Part model, mm, in its own coordinate system. A direction names the side the tool comes from. Coordinates: 2 decimals unless noted, no trailing zeros. Write each loop counter-clockwise with the first axis right and the second up, starting at its lowest first coordinate (ties: lowest second). Pieces come first, ordered by that corner, then holes. Notation, with made-up numbers: (-36.75, 70) - (14.25, 70) arc R19 cw to (14.25, 87) - close; hole circle Ø7 at (25, -20.5). An arc over 180 degrees is marked (long way). Use a Markdown table: item, result.
```python
from build123d import *

# Parameters (mm, degrees)
F0_R     = 7.9375
F0_R_2   = 11.828435
F0_R_3   = 12.7
F0_R_4   = 6.35
F1_DEPTH = 12.7


with BuildPart() as f1:
    # F0 (on Front) → F1 (new body)
    with BuildSketch(Plane.XZ):
        with BuildLine():
            Line((82.55, 7.45639), (82.55, 34.925))
            ThreePointArc((82.55, 34.925), (50.8, 66.675), (19.05, 34.925))
            Line((19.05, 34.925), (19.05, 33.3375))
            ThreePointArc((19.05, 33.3375), (17.655096, 29.969904), (14.2875, 28.575))
            Line((14.2875, 28.575), (-14.2875, 28.575))
            ThreePointArc((-14.2875, 28.575), (-17.655096, 29.969904), (-19.05, 33.3375))
            Line((-19.05, 33.3375), (-19.05, 34.925))
            ThreePointArc((-19.05, 34.925), (-50.8, 66.675), (-82.55, 34.925))
            Line((-82.55, 34.925), (-82.55, 7.45639))
            ThreePointArc((-82.55, 7.45639), (-83.623483, 4.44432), (-86.36, 2.790112))
            ThreePointArc((-86.36, 2.790112), (-101.503534, -17.789696), (-82.55, -34.925))
            Line((-82.55, -34.925), (-53.975, -34.925))
            ThreePointArc((-53.975, -34.925), (-47.239808, -37.714808), (-44.45, -44.45))
            Line((-44.45, -44.45), (-44.45, -51.575074))
            ThreePointArc((-44.45, -51.575074), (-41.660192, -58.310266), (-34.925, -61.100074))
            Line((-34.925, -61.100074), (-18.634955, -61.100074))
            Line((-18.634955, -61.100074), (-18.634955, -48.400074))
            ThreePointArc((-18.634955, -48.400074), (0.011654, -28.578944), (19.449271, -47.625))
            Line((19.449271, -47.625), (19.449271, -60.325))
            Line((19.449271, -60.325), (34.925, -60.325))
            ThreePointArc((34.925, -60.325), (41.660192, -57.535192), (44.45, -50.8))
            Line((44.45, -50.8), (44.45, -44.45))
            ThreePointArc((44.45, -44.45), (47.239808, -37.714808), (53.975, -34.925))
            Line((53.975, -34.925), (82.55, -34.925))
            ThreePointArc((82.55, -34.925), (101.503534, -17.789696), (86.36, 2.790112))
            ThreePointArc((86.36, 2.790112), (83.623483, 4.44432), (82.55, 7.45639))
        make_face()
        with Locations((-82.55, -15.875)):
            Circle(F0_R, mode=Mode.SUBTRACT)
        Circle(F0_R_2, mode=Mode.SUBTRACT)
        with Locations((82.55, -15.875)):
            Circle(F0_R, mode=Mode.SUBTRACT)
        with Locations((-50.8, 34.925)):
            Circle(F0_R_3, mode=Mode.SUBTRACT)
        with Locations((50.8, 34.925)):
            Circle(F0_R_3, mode=Mode.SUBTRACT)
        with Locations((-82.55, -15.875)):
            Circle(F0_R)
        with Locations((-82.55, -15.875)):
            Circle(F0_R_4, mode=Mode.SUBTRACT)
        with Locations((82.55, -15.875)):
            Circle(F0_R)
        with Locations((82.55, -15.875)):
            Circle(F0_R_4, mode=Mode.SUBTRACT)
    extrude(amount=F1_DEPTH)


solid = f1.part
```
Item 1: Drop flat-ended pins along their axis: P1, Ø2, axis at y = -11.5, z = -41.5, coming from the -X side; P2, Ø4, axis at x = -67.5, y = -3.5, coming from the -Z side (3 decimals); P3, Ø12, axis at x = 75.5, z = 47.5, coming from the +Y side; P4, Ø15, axis at x = -50.8, z = 34.925, coming from the +Y side. Give the stop position or say it passes through.
From the geometry:
| item | result |
|---|---|
| P1 | x = -45.31 |
| P2 | z = -34.925 |
| P3 | y = 0 |
| P4 | through |
Item 2: Band-saw the part on D-D, the plane y = -4.5. Count the separate pieces of the cut face and the enclosed holes in it, then the cut area to 3 significant figures.
From the geometry:
| item | result |
|---|---|
| separate pieces | 1 |
| enclosed holes | 5 |
| area | 15,100 mm^2 |
Item 3: Band-saw the part on B-B, the plane x = 50.8. Give the cut face in (y, z) (3 decimals), then the cut area to 3 significant figures.
From the geometry:
| item | result |
|---|---|
| outline | (-12.7, -35.47) - (0, -35.47) - (0, 22.225) - (-12.7, 22.225) - close; (-12.7, 47.625) - (0, 47.625) - (0, 66.675) - (-12.7, 66.675) - close |
| area | 975 mm^2 |
Item 4: Band-saw the part on C-C, the plane z = -33. Give the cut face in (x, y).
From the geometry:
| item | result |
|---|---|
| outline | (-90.89, -12.7) - (-11.81, -12.7) - (-11.81, 0) - (-90.89, 0) - close; (12.61, -12.7) - (90.89, -12.7) - (90.89, 0) - (12.61, 0) - close |
Item 5: Drill centre lines: probe 1 along X at (y, z) = (-11.25, 41.5); probe 2 along X at (y, z) = (-3.25, -50); probe 3 along Z at (x, y) = (0, -6.5) (3 decimals). Where is each one in solid material? Low to high.
From the geometry:
| item | result |
|---|---|
| probe 1 | -81.86 to -61.67, -39.93 to -19.74, 19.74 to 39.93, 61.67 to 81.86 |
| probe 2 | -44.45 to -18.63, 19.45 to 44.45 |
| probe 3 | -28.579 to -11.828, 11.828 to 28.575 |
Item 6: Band-saw the part on A-A, the plane z = -20. Give the cut face in (x, y), then the cut area to 3 significant figures.
From the geometry:
| item | result |
|---|---|
| outline | (-101.15, -12.7) - (-87.38, -12.7) - (-87.38, 0) - (-101.15, 0) - close; (-77.72, -12.7) - (77.72, -12.7) - (77.72, 0) - (-77.72, 0) - close; (87.38, -12.7) - (101.15, -12.7) - (101.15, 0) - (87.38, 0) - close |
| area | 2,320 mm^2 |
Item 7: Two-plate mould, pull along X, no slides. Class faces 1 (the face through (-1, 0, 18)), 2 (the face through (76.206, -6.261, -15.596)), 3 (the face through (-41.73, -6.26, -58.24)), 4 (the face through (47.166, -6.261, -37.789)): pulls with the +X half, pulls with the -X half, needs draft (parallel to the pull), parting line crosses it, or undercut.
From the geometry:
| item | result |
|---|---|
| face 1 | needs draft |
| face 2 | undercut |
| face 3 | pulls with the -X half |
| face 4 | pulls with the +X half |
Item 8: Which spindle directions (+Z, -Z, +X, -X, +Y, -Y) get a long thin tool onto all of the face, cutting with end or side? Do faces 5 (the face through (0, -6, 28.575)), 6 (the face through (-44.45, -6, -48)), 7 (the face through (-18.635, -6, -55)), 8 (the face through (44.45, -6, -48)). Say none if no direction does.
From the geometry:
| item | result |
|---|---|
| face 5 | +Z, +Y, -Y |
| face 6 | -Z, -X, +Y, -Y |
| face 7 | -Z, +Y, -Y |
| face 8 | -Z, +X, +Y, -Y |
